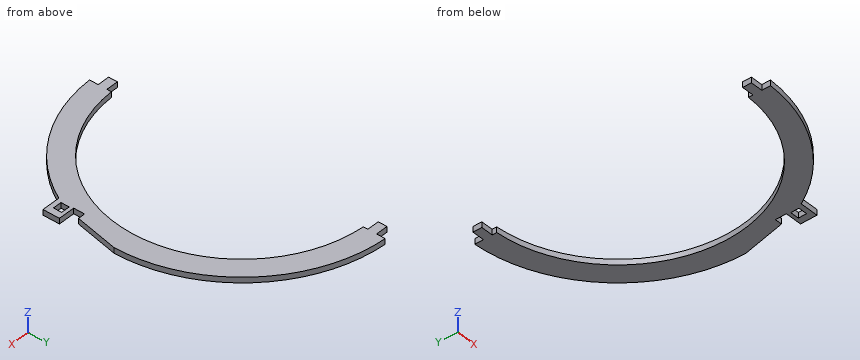
Autodesk Inventor part; units mm, degrees
ref_plane "YZ Plane" through (0, 0, 0) normal (1, 0, 0) x (0, 1, 0)
ref_plane "XZ Plane" through (0, 0, 0) normal (0, 1, 0) x (-1, 0, 0)
ref_plane "XY Plane" through (0, 0, 0) normal (0, 0, 1) x (1, 0, 0)
sketch "Sketch1" plane through (0, 0, 0) normal (0, 0, 1) x (1, 0, 0)
  arc A0 (0, -146.05) -> (0, 146.05) centre (0, 0) ccw
  line L0 (0, 0) -> (0, 226.0912) construction
  line L1 (0, 226.0912) -> (0, -237.3269) construction
  line L2 (6.35, 145.9119) -> (6.35, 171.3324)
  line L3 (6.35, -145.9119) -> (6.35, -171.3324)
  line L4 (0, 146.05) -> (0, 151.13)
  line L5 (0, 151.13) -> (6.35, 151.13)
  line L6 (6.35, 151.13) -> (-7.62, 151.13)
  line L7 (-7.62, 151.13) -> (-7.62, 161.29)
  line L8 (-7.62, 161.29) -> (6.35, 161.29)
  line L9 (0, -146.05) -> (0, -151.13)
  line L10 (0, -151.13) -> (6.35, -151.13)
  line L11 (6.35, -151.13) -> (-7.62, -151.13)
  line L12 (-7.62, -151.13) -> (-7.62, -161.29)
  line L13 (-7.62, -161.29) -> (6.35, -161.29)
  line L14 (171.45, 0) -> (171.45, -82.55)
  line L15 (171.45, -82.55) -> (150.2684, -82.55)
  arc A1 (0, -171.45) -> (150.2684, -82.55) centre (0, 0) ccw
  arc A2 (171.45, 0) -> (0, 171.45) centre (0, 0) ccw
  dimension "d20" = 292.1
  dimension "d21" = 6.35
  dimension "d22" = 6.35
  dimension "d23" = 5.08
  dimension "d24" = 13.97
  dimension "d25" = 10.16
  dimension "d26" = 5.08
  dimension "d27" = 13.97
  dimension "d28" = 10.16
  dimension "d29" = 82.55
  dimension "d45" = 171.45
  dimension "d46" = 171.45
ref_plane "Work Plane1" through (0, 0, 6.35) normal (0, 0, 1) x (1, 0, 0)
sketch "Sketch2" plane through (0, 0, 6.35) normal (0, 0, 1) x (1, 0, 0)
  line L0 (171.45, -82.55) -> (171.45, 0)
  line L1 (171.45, -82.55) -> (171.45, -77.0382) construction
  line L2 (171.45, -77.0382) -> (163.83, -77.0382) construction
  line L3 (163.83, -77.0382) -> (153.67, -77.0382)
  line L4 (153.67, -77.0382) -> (153.67, -67.5132)
  line L5 (153.67, -67.5132) -> (163.83, -67.5132)
  line L6 (163.83, -67.5132) -> (163.83, -77.0382)
  line L7 (171.45, 0) -> (171.45, -63.5) construction
  line L8 (171.45, -63.5) -> (152.4, -63.5)
  line L9 (152.4, -63.5) -> (152.4, -50.8)
  line L10 (152.4, -50.8) -> (160.5643, -50.8)
  arc A0 (171.45, 0) -> (6.35, 171.3324) centre (0, 0) ccw
  line L11 (160.5643, -50.8) -> (171.45, 0)
  line L12 (171.45, 0) -> (171.45, -63.5)
  point P0 (171.45, -44.45)
  dimension "d32" = 5.5118
  dimension "d33" = 7.62
  dimension "d34" = 10.16
  dimension "d35" = 9.525
  dimension "d38" = 63.5
  dimension "d39" = 19.05
  dimension "d40" = 12.7
  dimension "d44" = 102.095
extrude "Extrusion5" add sketch "Sketch1" along normal blind 6.35 contours A0 L2 A2 L14 L15 A1 L3 | L10 L3 L13 L12 L11 | L5 L6 L7 L8 L2
extrude "Extrusion6" cut sketch "Sketch2" against normal blind 6.35
properties part number "MiddleHoop"
Read the model definition and answer for the solid it produces. Units are mm, in the model's axes. Coordinates: 2 decimals unless noted, no trailing zeros. Write each loop counter-clockwise with the first axis right and the second up, starting at its lowest first coordinate (ties: lowest second). Pieces come first, ordered by that corner, then holes. Notation, with made-up numbers: (38, 54) -> (57, 54) arc R22 ccw to (57, 66) -> close; hole circle Ø6 at (86, 54). An arc over 180 degrees is marked (long way). Answer as a JSON object with one key per item and string values.
Q1. The part is cut by section C-C on x = 46. Give the vertices of the cut face in (y, z).
The answers:
{"outline": "(-165.16, 0) -> (-138.62, 0) -> (-138.62, 6.35) -> (-165.16, 6.35) -> close; (138.62, 0) -> (165.16, 0) -> (165.16, 6.35) -> (138.62, 6.35) -> close"}
Q2. Consider line 1 (Y direction, x = 27.5, z = 4.25); line 2 (Y direction, x = 132, z = 1.5); line 3 (X direction, y = -30, z = 1.75). Determine where each line is inside the solid, lowest interval first. Write a range as [from, to].
The answers:
{"line 1": "y = [-169.23, -143.44], [143.44, 169.23]", "line 2": "y = [-109.41, -62.5], [62.5, 109.41]", "line 3": "x = [142.94, 165.02]"}
Q3. Flat-ended cylindrical pins translate along their axes: pin 1 Ø1.5 at (y, z) = (-17.5, 2) entering from +X; pin 2 Ø3 at (x, z) = (160.5, 2.5) entering from -Y; pin 3 Ø1.9 at (x, z) = (0.5, 2.5) entering from +Y. Find the tip coordinate at first contact, or state that the pin passes through.
The answers:
{"pin 1": "stops at x = 167.86", "pin 2": "stops at y = -82.55", "pin 3": "stops at y = 161.29"}
Q4. The part is cut by section A-A on x = 0. Give the vertices of the cut face in (y, z).
The answers:
{"outline": "(-161.29, 0) -> (-151.13, 0) -> (-151.13, 6.35) -> (-161.29, 6.35) -> close; (151.13, 0) -> (161.29, 0) -> (161.29, 6.35) -> (151.13, 6.35) -> close"}
Q5. The part is cut by section B-B on z = 1.75. Give the vertices of the cut face in (x, y), then the cut area to 3 significant figures.
The answers:
{"outline": "(-7.62, -161.29) -> (6.35, -161.29) -> (6.35, -171.33) arc R171.45 ccw to (150.27, -82.55) -> (171.45, -82.55) -> (171.45, -63.5) -> (152.4, -63.5) -> (152.4, -50.8) -> (160.56, -50.8) -> (171.45, 0) arc R171.45 ccw to (6.35, 171.33) -> (6.35, 161.29) -> (-7.62, 161.29) -> (-7.62, 151.13) -> (6.35, 151.13) -> (6.35, 145.91) arc R146.05 cw to (6.35, -145.91) -> (6.35, -151.13) -> (-7.62, -151.13) -> close; hole (153.67, -77.04) -> (163.83, -77.04) -> (163.83, -67.51) -> (153.67, -67.51) -> close", "area": "12,600 mm2"}
Q6. The part is cut by section D-D on y = -23.5. Give the vertices of the cut face in (x, z), then the cut area to 3 significant figures.
The answers:
{"outline": "(144.15, 0) -> (166.41, 0) -> (166.41, 6.35) -> (144.15, 6.35) -> close", "area": "141 mm2"}
